Verification items for the finished model (mm, model axes). Face numbers are marked on the shaded views. A direction names the side the tool comes from. Coordinates: 2 decimals unless noted, no trailing zeros. Write each loop counter-clockwise with the first axis right and the second up, starting at its lowest first coordinate (ties: lowest second). Pieces come first, ordered by that corner, then holes. Notation, with made-up numbers: (7, -17) - (19, -17) arc R31 ccw to (19, 22) - close; hole circle Ø1 at (50, -8.5). An arc over 180 degrees is marked (long way). Use one line per item in the form item = value. Start each with the question number.
(1) Sectioned sample at A-A (x = -3.25). Record the cut outline in (y, z), and give its area (3 significant figures).
(2) Sectioned sample at B-B (y = 21.5). Record the cut outline in (x, z), and give its area (3 significant figures).
(3) Mould release check, pull along Y, two halves, no side actions. Record for the marked faces 4, 5, 6 and 7: released by +Y, released by -Y, zero draft, split by the parting line, or undercut.
(4) Sectioned sample at D-D (y = -23). Record the cut outline in (x, z), and give its area (3 significant figures).
(5) Material ranges on line 1 (X direction, y = -10, z = 0.3); line 2 (Y direction, x = 2.5, z = 1.5); line 3 (X direction, y = 17, z = 2.7), recorded low to high. Write a range as [from, to].
(6) Tool access check on the marked faces 1, 2 and 3. Record the directions out of +Z, -Z, +X, -X, +Y, -Y that give a thin tool (end or side, any length) a straight path to the whole face; none if there is none.
from build123d import *

# Parameters (mm, degrees)
SKETCH_1_W          = 22
SKETCH_1_H          = 60
EXTRUDE_2_DEPTH     = 3
SKETCH_2_W          = 4
SKETCH_2_H          = 5
CUT_EXTRUDE_1_DEPTH = 5
FILLET_1_R          = 4


with BuildPart() as part:
    # Эскиз1 → Бобышка-Вытянуть2 (new body)
    with BuildSketch(Plane.XY):
        Rectangle(SKETCH_1_W, SKETCH_1_H)
        Polygon((4, 26), (-4, 26), (-4, 2), (-7, 2), (-7, -26), (7, -26), (7, 2), (4, 2), align=None, mode=Mode.SUBTRACT)
    extrude(amount=EXTRUDE_2_DEPTH)

    # Эскиз2 → Вырез-Вытянуть1 (cut)
    with BuildSketch(Plane.XY.offset(3)):
        with Locations((-9, -23.5)):
            Rectangle(SKETCH_2_W, SKETCH_2_H)
    extrude(amount=-CUT_EXTRUDE_1_DEPTH, mode=Mode.SUBTRACT)

    # Скругление1
    fillet_1_edges = [part.edges().sort_by_distance(p)[0] for p in [
        (-11, 30, 1.5),
        (11, 30, 1.5),
        (11, -30, 1.5),
        (-11, -30, 1.5),
    ]]
    fillet(fillet_1_edges, radius=FILLET_1_R - 0.0001)  # a hair under: the kernel refuses the full size


solid = part.part
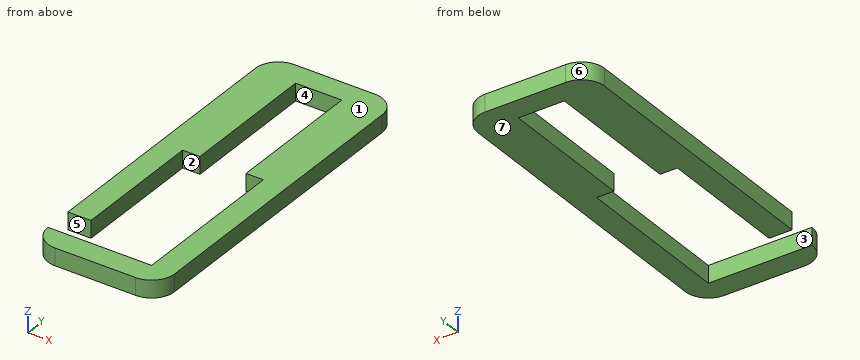
Answers below:
q1.outline = (-30, 0) - (-26, 0) - (-26, 3) - (-30, 3) - close; (26, 0) - (30, 0) - (30, 3) - (26, 3) - close
q1.area = 24.0 mm2
q2.outline = (-11, 0) - (-4, 0) - (-4, 3) - (-11, 3) - close; (4, 0) - (11, 0) - (11, 3) - (4, 3) - close
q2.area = 42.0 mm2
q3.face_4 = undercut
q3.face_5 = undercut
q3.face_6 = released by +Y
q3.face_7 = zero draft
q4.outline = (7, 0) - (11, 0) - (11, 3) - (7, 3) - close
q4.area = 12.0 mm2
q5.line_1 = [-11, -7], [7, 11]
q5.line_2 = [-30, -26], [26, 30]
q5.line_3 = [-11, -4], [4, 11]
q6.face_1 = +Z, +X, -X, +Y, -Y
q6.face_2 = +Z, -Z
q6.face_3 = +Z, -Z, -X
